Could you check a few things on this model? Use its own coordinates, in mm. A direction names the side the tool comes from. Round coordinates to 2 decimals unless told otherwise and drop trailing zeros. Loops run counter-clockwise (first coordinate to the right, second up) from the corner with the lowest first, then second, coordinate; pieces in that order, holes last.
Autodesk Inventor part; units mm, degrees
ref_plane "Work Plane4" through (-4.0321, -4.1704, -0.5659) normal (-0.7071, -0.7071, 0) x (0.204, -0.204, 0.9575)
ref_plane "YZ Plane" through (0, 0, 0) normal (1, 0, 0) x (0, 1, 0)
ref_plane "XZ Plane" through (0, 0, 0) normal (0, 1, 0) x (-1, 0, 0)
sketch "Sketch1" plane through (0, 0, 0) normal (0, 0, 1) x (1, 0, 0)
  line L0 (-16.9, 21.4) -> (-16.9, 16.9) construction
  arc A0 (-22.9, 19.9) -> (-19.9, 22.9) centre (-19.9, 19.9) ccw construction
  line L1 (-16.9, 16.9) -> (16.9, 16.9) construction
  line L2 (16.9, 16.9) -> (16.9, -16.9) construction
  line L3 (16.9, -16.9) -> (-16.9, -16.9) construction
  line L4 (-16.9, -16.9) -> (-16.9, 16.9) construction
  arc A1 (22.9, -19.9) -> (19.9, -22.9) centre (19.9, -19.9) ccw construction
  line L5 (22.9, 19.9) -> (22.9, -19.9) construction
  arc A2 (19.9, 22.9) -> (22.9, 19.9) centre (19.9, 19.9) ccw construction
  line L6 (-19.9, 22.9) -> (19.9, 22.9) construction
  arc A3 (-22.9, 19.9) -> (-19.9, 22.9) centre (-19.9, 19.9) ccw construction
  line L7 (-22.9, -19.9) -> (-22.9, 19.9) construction
  arc A4 (-19.9, -22.9) -> (-22.9, -19.9) centre (-19.9, -19.9) ccw construction
  line L8 (19.9, -22.9) -> (-19.9, -22.9) construction
  line L9 (-21.4, 16.9) -> (-16.9, 16.9) construction
  line L10 (-16.9, -16.9) -> (-21.4, -16.9) construction
  line L11 (-16.9, -16.9) -> (-16.9, -21.4) construction
  line L12 (16.9, -21.4) -> (16.9, -16.9) construction
  line L13 (21.4, -16.9) -> (16.9, -16.9) construction
  line L14 (16.9, 16.9) -> (21.4, 16.9) construction
  line L15 (16.9, 16.9) -> (16.9, 21.4) construction
  line L16 (-16.8009, 21.2415) -> (21.2415, -16.8009)
  line L17 (21.2415, -16.8009) -> (16.8009, -21.2415)
  line L18 (16.8009, -21.2415) -> (-21.2415, 16.8009)
  line L19 (-21.2415, 16.8009) -> (-16.8009, 21.2415)
  line L20 (-16.8009, 21.2415) -> (16.8009, -21.2415) construction
  line L21 (21.2415, -16.8009) -> (-21.2415, 16.8009) construction
  line L22 (-16.8009, 21.2415) -> (36.9991, 21.2415) construction
  line L23 (-21.2415, 16.8009) -> (-22.9, 16.8009)
  line L24 (16.8009, -21.2415) -> (16.8009, -22.9)
  line L25 (16.8009, -22.9) -> (-22.9, 16.8009)
  line L26 (-16.8009, 21.2415) -> (-16.8009, 22.9)
  line L27 (21.2415, -16.8009) -> (22.9, -16.8009)
  line L28 (22.9, -16.8009) -> (-16.8009, 22.9)
  line L29 (-22.9, 16.8009) -> (-22.9, 11.5863)
  line L30 (16.8009, -22.9) -> (11.5863, -22.9)
  line L31 (-22.9, 11.5863) -> (11.5863, -22.9)
  point P0 (0, 0)
  dimension "d0" = 53.8
  dimension "d1" = 45
  dimension "d2" = 6.28
  dimension "d5" = 8
extrude "Extrusion1" add sketch "Sketch1" along normal blind 30
ref_plane "Work Plane1" through (16.9, -16.9, -8) normal (-0.7071, -0.7071, 0) x (0, 0, 1)
sketch "Sketch7" plane through (0, 0, 30) normal (0, 0, 1) x (1, 0, 0)
  line L0 (21.2415, -16.8009) -> (22.9, -16.8009)
  line L1 (22.9, -16.8009) -> (-16.8009, 22.9)
  line L2 (-16.8009, 22.9) -> (-16.8009, 21.2415)
  line L3 (-16.8009, 21.2415) -> (-21.2415, 16.8009)
  line L4 (-21.2415, 16.8009) -> (-22.9, 16.8009)
  line L5 (-22.9, 16.8009) -> (-22.9, 11.5863)
  line L6 (-22.9, 11.5863) -> (11.5863, -22.9)
  line L7 (11.5863, -22.9) -> (16.8009, -22.9)
  line L8 (16.8009, -22.9) -> (16.8009, -21.2415)
  line L9 (16.8009, -21.2415) -> (21.2415, -16.8009)
  line L10 (3.0496, 3.0496) -> (-5.6569, -5.6569)
  line L11 (-22.9, 11.5863) -> (11.5863, -22.9)
  line L12 (17.9785, -3.9418) -> (10.0409, -11.8794)
  line L13 (10.0409, -11.8794) -> (-11.8794, 10.0409)
  line L14 (-11.8794, 10.0409) -> (-3.9418, 17.9785)
  line L15 (-3.9418, 17.9785) -> (17.9785, -3.9418)
  line L16 (17.9785, -3.9418) -> (-11.8794, 10.0409) construction
  line L17 (10.0409, -11.8794) -> (-3.9418, 17.9785) construction
  line L18 (-11.8794, 10.0409) -> (-11.8794, 17.9785)
  line L19 (22.9, -16.8009) -> (-16.8009, 22.9)
  line L20 (10.0409, -11.8794) -> (17.9785, -11.8794)
  point P0 (0, 0)
  dimension "d28" = 31
  dimension "d29" = 1.3
extrude "Extrusion7" cut sketch "Sketch7" against normal through all contours L20 L12 L1 | L12 L13 L10 L1 | L1 L14 L15 L12 | L10 L13 L14 L1 | L14 L18 L1
sketch "Sketch13" plane through (0, 0, 30) normal (0, 0, 1) x (1, 0, 0)
  line L0 (-11.8794, 10.0409) -> (-11.8794, 17.9785) construction
  line L1 (-11.8794, 17.9785) -> (-16.8009, 22.9) construction
  line L2 (-16.8009, 22.9) -> (-16.8009, 21.2415)
  line L3 (-16.8009, 21.2415) -> (-21.2415, 16.8009)
  line L4 (-21.2415, 16.8009) -> (-22.9, 16.8009)
  line L5 (-22.9, 16.8009) -> (-22.9, 11.5863) construction
  line L6 (-22.9, 11.5863) -> (11.5863, -22.9) construction
  line L7 (11.5863, -22.9) -> (16.8009, -22.9) construction
  line L8 (16.8009, -22.9) -> (16.8009, -21.2415)
  line L9 (16.8009, -21.2415) -> (21.2415, -16.8009)
  line L10 (21.2415, -16.8009) -> (22.9, -16.8009)
  line L11 (22.9, -16.8009) -> (17.9785, -11.8794) construction
  line L12 (17.9785, -11.8794) -> (10.0409, -11.8794) construction
  line L13 (10.0409, -11.8794) -> (-11.8794, 10.0409) construction
  line L14 (-11.7794, 10.0823) -> (-11.7794, 18.02) construction
  line L15 (-11.7794, 18.02) -> (-16.9009, 23.1414) construction
  line L16 (-16.9009, 23.1414) -> (-16.9009, 21.2829)
  line L17 (-16.9009, 21.2829) -> (-21.2829, 16.9009)
  line L18 (-21.2829, 16.9009) -> (-23, 16.9009)
  line L19 (-23, 16.9009) -> (-23, 11.5449) construction
  line L20 (-23, 11.5449) -> (11.5449, -23) construction
  line L21 (11.5449, -23) -> (16.9009, -23) construction
  line L22 (16.9009, -23) -> (16.9009, -21.2829)
  line L23 (16.9009, -21.2829) -> (21.2829, -16.9009)
  line L24 (21.2829, -16.9009) -> (23.1414, -16.9009)
  line L25 (23.1414, -16.9009) -> (18.02, -11.7794) construction
  line L26 (18.02, -11.7794) -> (10.0823, -11.7794) construction
  line L27 (10.0823, -11.7794) -> (-11.7794, 10.0823) construction
  line L28 (16.8009, -22.9) -> (16.9009, -22.9)
  line L29 (22.9, -16.8009) -> (23, -16.9009)
  line L30 (-21.2415, 16.8009) -> (-22.9, 16.8009)
  line L31 (-22.9, 16.8009) -> (-22.9, 16.9009)
  line L32 (-16.8009, 22.9) -> (-16.9009, 23)
  point P0 (0, 0)
  dimension "d65" = 0.1
extrude "IM_offset" add sketch "Sketch13" against normal up to surface (30 mm away)
sketch "Sketch14" plane through (-11.8794, 10.0409, 0) normal (0.7071, 0.7071, 0) x (-0.7071, 0.7071, 0)
  circle A0 centre (-15.5978, 14.947) radius 12.7
  circle A1 centre (-15.5978, 14.947) radius 12.9
  point P0 (-15.5, 0)
  dimension "d68" = 0.2
ref_plane "Work Plane4" through (-4.0321, -4.1704, -0.5659) normal (-0.7071, -0.7071, 0) x (0.204, -0.204, 0.9575)
extrude "Extrusion11" cut sketch "Sketch14" against normal up to surface (4.5 mm away) contours A0 | A1
sketch "Sketch15" plane through (-4.0321, -4.1704, 14.947) normal (0.7071, 0.7071, 0) x (0, 0, -1)
  circle A0 centre (0, 0) radius 12.45
  circle A1 centre (0, 0) radius 10.1726
  point P0 (14.947, 0.0978)
extrude "Extrusion12" cut sketch "Sketch15" against normal through all contours A1
equation "\"d3\" = MirrorThickness1"
equation "\"MirrorThickness1\" = 30"
properties part number "20_Cube_Insert_Mirror_Holder_wLogo_v3"
Item 1: We'd pull the mould along X, two halves only. Please class faces 4 (the cylindrical face through (-1.232, -3.745, 27.737)), 5 (the flat face through (20.5, -14.4, 14.8)), 6 (the flat face through (-2, -2, 0)): released by +X, released by -X, zero draft, split by the parting line, or undercut.
Results list:
face 4: undercut
face 5: released by +X
face 6: zero draft
Item 2: If we section it at B-B, the plane z = 10: Please give me the cut outline in (x, y), then the cut area to 3 significant figures.
Results list:
outline: (-22.9, 11.59) - (-11.87, 0.56) - (-10.32, 2.11) - (-12.46, 4.25) - (-9.27, 7.44) - (-11.88, 10.04) - (-11.88, 17.98) - (-16.9, 23) - (-16.9, 21.28) - (-21.28, 16.9) - (-22.9, 16.9) - close; (0.7, -12.01) - (11.59, -22.9) - (16.9, -22.9) - (16.9, -21.28) - (21.28, -16.9) - (23, -16.9) - (17.98, -11.88) - (10.04, -11.88) - (7.57, -9.41) - (4.39, -12.6) - (2.25, -10.46) - close
area: 310 mm2
Item 3: For faces 1 (the flat face through (2.766, -10.971, 11.185)), 2 (the flat face through (-16.901, 22, 15)), 3 (the flat face through (14, -11.879, 15)), which set-ups out of +Z, -Z, +X, -X, +Y, -Y let a thin tool reach every point of the face, with its end or its side?
Results list:
face 1: none
face 2: +Z, -Z, -X, +Y
face 3: +Z, -Z, +X, +Y
Item 4: If we section it at A-A, the plane z = 6.5: Please give me the cut outline in (x, y).
Results list:
outline: (-22.9, 11.59) - (-9.6, -1.72) - (-8.04, -0.16) - (-10.93, 2.72) - (-7.74, 5.91) - (-11.88, 10.04) - (-11.88, 17.98) - (-16.9, 23) - (-16.9, 21.28) - (-21.28, 16.9) - (-22.9, 16.9) - close; (-1.58, -9.73) - (11.59, -22.9) - (16.9, -22.9) - (16.9, -21.28) - (21.28, -16.9) - (23, -16.9) - (17.98, -11.88) - (10.04, -11.88) - (6.04, -7.88) - (2.86, -11.07) - (-0.03, -8.18) - close
Item 5: If we section it at C-C, the plane y = 15: Please give me the cut outline in (x, z).
Results list:
outline: (-22.9, 0) - (-11.88, 0) - (-11.88, 30) - (-22.9, 30) - close
Item 6: If we section it at D-D, the plane x = 9: Please give me the cut outline in (y, z).
Results list:
outline: (-20.31, 0) - (-10.84, 0) - (-10.84, 30) - (-20.31, 30) - close
Item 7: Will these pins go through, and if not, where does the flat tip stop? pin 1 (2 mm diameter, centred on y = -5.5, z = 22, fed in from -X); pin 2 (8.5 mm diameter, centred on y = 12.5, z = 15.5, fed in from +X); pin 3 (2 mm diameter, centred on x = 18, z = 21.5, fed in from +Y); pin 4 (4 mm diameter, centred on x = -8.5, z = 16.5, fed in from -Y) (3 decimals).
Results list:
pin 1: passes through
pin 2: stops at x = -10.09
pin 3: stops at y = -11.88
pin 4: stops at y = 7.435
Item 8: If I drill on line 1 along X through (y, z) = (15, 6.25); line 2 along X through (y, z) = (-4, 28), over which ranges is the centre line in solid material (lowest first)?
Results list:
line 1: x = -22.9 to -11.88
line 2: x = -7.31 to 2.16
